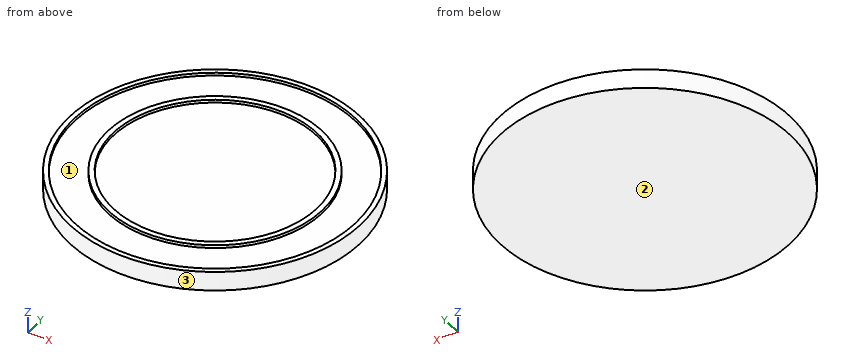
```python
from build123d import *

# Parameters (mm, degrees)
SKETCH_R        = 150
PAD_DEPTH       = 20
SKETCH001_R     = 145
SKETCH001_R_2   = 110.45
POCKET_DEPTH    = 3
SKETCH002_R     = 105
POCKET001_DEPTH = 3


with BuildPart() as part:
    # Sketch → Pad (new body)
    with BuildSketch(Plane.XY):
        Circle(SKETCH_R)
    extrude(amount=-PAD_DEPTH)

    # Sketch001 → Pocket (cut)
    with BuildSketch(Plane.XY):
        Circle(SKETCH001_R)
        Circle(SKETCH001_R_2, mode=Mode.SUBTRACT)
    extrude(amount=-POCKET_DEPTH, mode=Mode.SUBTRACT)

    # Sketch002 → Pocket001 (cut)
    with BuildSketch(Plane.XY):
        Circle(SKETCH002_R)
    extrude(amount=-POCKET001_DEPTH, mode=Mode.SUBTRACT)


solid = part.part
```
Could you check a few things on this model? Use its own coordinates, in mm. Face numbers are marked on the shaded views. Round coordinates to 2 decimals unless told otherwise and drop trailing zeros. Loops run counter-clockwise (first coordinate to the right, second up) from the corner with the lowest first, then second, coordinate; pieces in that order, holes last. Notation, with made-up numbers: M 22,-36.75 L 78,-36.75 A11 cw 78,-16.75 Z; hole C 3.5,22.5 d4. An arc over 180 degrees is marked long. Write item = value, one per line.
1. I want a section at B-B, the plane y = 0. Write out the boundary of the cut face in (x, z), and give its area (3 significant figures).
Results below:
outline = M -150,-20 L 150,-20 L 150,0 L 145,0 L 145,-3 L 110.45,-3 L 110.45,0 L 105,0 L 105,-3 L -105,-3 L -105,0 L -110.45,0 L -110.45,-3 L -145,-3 L -145,0 L -150,0 Z
area = 5,160 mm²
2. Will these pins go through, and if not, where does the flat tip stop? P1, Ø2, axis at x = 83.5, z = -6.5, coming from the -Y side; P2, Ø1, axis at x = -38.5, z = -9.5, coming from the +Y side; P3, Ø6, axis at x = 98.5, z = -11, coming from the +Y side.
Results below:
P1 = -125.27
P2 = 145.11
P3 = 115.67
3. I want a section at A-A, the plane x = -97.5. Write out the boundary of the cut face in (y, z).
Results below:
outline = M -113.99,-20 L 113.99,-20 L 113.99,0 L 107.33,0 L 107.33,-3 L 51.89,-3 L 51.89,0 L 38.97,0 L 38.97,-3 L -38.97,-3 L -38.97,0 L -51.89,0 L -51.89,-3 L -107.33,-3 L -107.33,0 L -113.99,0 Z
4. Thinking about a two-plate mould opening in Y: for the marked faces 1, 2 and 3, which applies, +Y half, -Y half, draft (parallel to the pull), parting line (faces both ways), or undercut?
Results below:
face_1 = undercut
face_2 = draft
face_3 = parting line
5. I need wall thicknesses on probe 1 along Y at (x, z) = (0, -0.9); probe 2 along Y at (x, z) = (53.5, -1.75); probe 3 along Z at (x, y) = (-127.5, -37). Which ranges of each line are inside material? Lowest first, please.
Results below:
probe_1 = -150 to -145, -110.45 to -105, 105 to 110.45, 145 to 150
probe_2 = -140.13 to -134.77, -96.63 to -90.35, 90.35 to 96.63, 134.77 to 140.13
probe_3 = -20 to -3
6. I want a section at C-C, the plane z = -8.5. Write out the boundary of the cut face in (x, y).
Results below:
outline = C 0,0 d300
7. I want a section at D-D, the plane y = -116.5. Write out the boundary of the cut face in (x, z).
Results below:
outline = M -94.49,-20 L 94.49,-20 L 94.49,0 L 86.33,0 L 86.33,-3 L -86.33,-3 L -86.33,0 L -94.49,0 Z
